Input: part model. Units: mm. Frame: model coordinates. Face numbers are marked on the shaded views. A direction names the side the tool comes from. Coordinates: 2 decimals unless noted, no trailing zeros. Write each loop counter-clockwise with the first axis right and the second up, starting at its lowest first coordinate (ties: lowest second). Pieces come first, ordered by that corner, then holes.
1) Section query B-B (y = 25). Output: boundary loops of the cut face in (x, z).
2) Line query: L1, parallel to Z at x = 2.5, y = 1.8; L2, parallel to X at y = 25, z = -3.6; L3, parallel to Z at x = 2.5, y = 4.25. Output: solid intervals per line, ascending.
3) Set-up query: the marked faces 5, 6, 7 and 8. Return all of +Z, -Z, +X, -X, +Y, -Y with unobstructed straight access to the full face (end or side cutting, diameter ignored); none if empty.
4) Draft query along X for the marked faces 1, 2, 3 and 4. Return one class per face: pulls with the +X half, pulls with the -X half, needs draft (parallel to the pull), parting line crosses it, or undercut.
5) Section query D-D (z = 22). Output: boundary loops of the cut face in (x, y), then the cut area to 3 significant figures.
6) Section query C-C (x = 2.5). State how many separate pieces and enclosed holes the cut face has, then the cut area to 3 significant figures.
7) Section query A-A (z = 18). Output: boundary loops of the cut face in (x, y), then the cut area to 3 significant figures.
8) Pin query (flat end, axial travel): pin 1 Ø4.5 at (x, z) = (-1, 11.5) entering from -Y; pin 2 Ø4 at (x, z) = (3, 0.5) entering from +Y; pin 3 Ø1 at (x, y) = (2.5, 8.5) entering from +Z. Return the tip coordinate at first contact, or that it passes through.
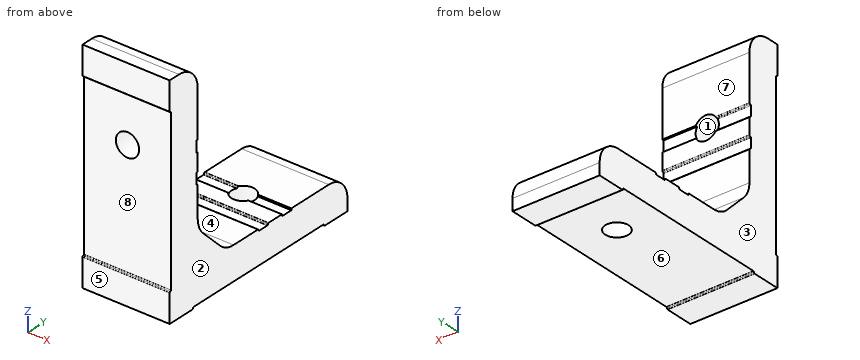
from build123d import *

# Parameters (mm, degrees)
ESBO_O1_W                  = 38
ESBO_O1_H                  = 38
RESSALTO_EXTRUS_O1_DEPTH   = 15
CORTE_EXTRUS_O1_DEPTH      = 52.28352562
ESBO_O7_W                  = 0.3
ESBO_O7_H                  = 28
ESBO_O7_W_2                = 28
ESBO_O7_H_2                = 0.3
ESBO_O7_W_3                = 2
ESBO_O7_H_3                = 2
CORTE_EXTRUS_O2_DEPTH      = 52.28352562
FURO_DE_DI_METRO_7_0_7_3_D = 4
FURO_DE_DI_METRO_7_0_7_2_D = 4
FILETE1_R                  = 4
FILETE2_R                  = 0.15


with BuildPart() as part:
    # Esboço1 → Ressalto-extrusão1 (new body)
    with BuildSketch(Plane(origin=(10, 0, 0), x_dir=(0, 0, -1), z_dir=(1, 0, 0))):
        with Locations((-12, 19)):
            Rectangle(ESBO_O1_W, ESBO_O1_H)
    extrude(amount=-RESSALTO_EXTRUS_O1_DEPTH)

    # Esboço2 → Corte-extrusão1 (cut, through all)
    with BuildSketch(Plane.ZY.offset(5)):
        Polygon((31, 38), (-1, 38), (-1, 12), (5, 6), (31, 6), align=None)
    extrude(amount=-CORTE_EXTRUS_O1_DEPTH, mode=Mode.SUBTRACT)

    # Esboço7 → Corte-extrusão2 (cut, through all)
    with BuildSketch(Plane(origin=(10, 0, 0), x_dir=(0, 0, -1), z_dir=(1, 0, 0))):
        with Locations((6.85, 19)):
            Rectangle(ESBO_O7_W, ESBO_O7_H)
        with Locations((-12, 0.15)):
            Rectangle(ESBO_O7_W_2, ESBO_O7_H_2)
        with Locations((-13, 5.85)):
            Rectangle(ESBO_O7_W_3, ESBO_O7_H_2)
        with Locations((1.15, 20)):
            Rectangle(ESBO_O7_W, ESBO_O7_H_3)
        with Locations((-18, 5.85)):
            Rectangle(ESBO_O7_W_3, ESBO_O7_H_2)
        with Locations((1.15, 25)):
            Rectangle(ESBO_O7_W, ESBO_O7_H_3)
    extrude(amount=-CORTE_EXTRUS_O2_DEPTH, mode=Mode.SUBTRACT)

    # Furo de diâmetro Ø7.0 (7)3 (through all)
    with Locations(Plane(origin=(0, 6, 0), x_dir=(1, 0, 0), z_dir=(0, 1, 0))):
        with Locations((2.5, -18)):
            Hole(FURO_DE_DI_METRO_7_0_7_3_D / 2)

    # Furo de diâmetro Ø7.0 (7)2 (through all)
    with Locations(Plane(origin=(0, 0, -7), x_dir=(-1, 0, 0), z_dir=(0, 0, -1))):
        with Locations((-2.5, 25)):
            Hole(FURO_DE_DI_METRO_7_0_7_2_D / 2)

    # Filete1
    filete1_edges = [part.edges().sort_by_distance(p)[0] for p in [
        (2.5, 6, 31),
        (2.5, 6, 5),
        (2.5, 12, -1),
        (2.5, 38, -1),
    ]]
    fillet(filete1_edges, radius=FILETE1_R)

    # Filete2
    filete2_edges = [part.edges().sort_by_distance(p)[0] for p in [
        (2.5, 5, -7),
        (2.5, 5, -6.7),
        (2.5, 33, -7),
        (2.5, 33, -6.7),
        (2.5, 0, 26),
        (2.5, 0.3, 26),
        (2.5, 0.3, -2),
        (2.5, 0, -2),
        (2.5, 19, -1.3),
        (2.5, 19, -1),
        (2.5, 21, -1.3),
        (2.5, 21, -1),
        (2.5, 5.7, 14),
        (2.5, 6, 14),
        (2.5, 5.7, 12),
        (2.5, 6, 12),
        (-2.116025404, 26, -1.3),
        (-2.116025404, 24, -1.3),
        (-2.116025404, 24, -1),
        (-2.116025404, 26, -1),
        (-2.116025404, 5.7, 19),
        (-2.116025404, 5.7, 17),
        (-2.116025404, 6, 17),
        (-2.116025404, 6, 19),
    ]]
    fillet(filete2_edges, radius=FILETE2_R - 0.0001)  # a hair under: the kernel refuses the full size


solid = part.part
Answer:
1. outline: (-5, -6.7) - (0.5, -6.7) - (0.5, -1.3) - (-5, -1.3) - close; (4.5, -6.7) - (10, -6.7) - (10, -1.3) - (4.5, -1.3) - close
2. L1: z = -7 to 16, 20 to 31
2. L2: x = -5 to 0.5, 4.5 to 10
2. L3: z = -7 to 16, 20 to 30.31
3. face 5: +Z, -Z, +X, -X, -Y
3. face 6: -Z, +X, -X
3. face 7: +Z, +X, -X, +Y
3. face 8: +X, -X, -Y
4. face 1: undercut
4. face 2: pulls with the +X half
4. face 3: pulls with the -X half
4. face 4: needs draft
5. outline: (-5, 0.3) - (10, 0.3) - (10, 6) - (-5, 6) - close
5. area: 85.5 mm2
6. separate pieces: 3
6. enclosed holes: 0
6. area: 368 mm2
7. outline: (-5, 0.3) - (0.5, 0.3) - (0.5, 5.7) - (-5, 5.7) - close; (4.5, 0.3) - (10, 0.3) - (10, 5.7) - (4.5, 5.7) - close
7. area: 59.4 mm2
8. pin 1: stops at y = 0.3
8. pin 2: stops at y = 35.94
8. pin 3: stops at z = 3
